Could you check a few things on this model? Use its own coordinates, in mm. A direction names the side the tool comes from. Round coordinates to 2 decimals unless told otherwise and drop trailing zeros. Write each loop counter-clockwise with the first axis right and the second up, starting at its lowest first coordinate (ties: lowest second). Pieces come first, ordered by that corner, then holes. Notation, with made-up numbers: (-8.5, -8.75) -> (-0.5, -8.75) arc R11 ccw to (-0.5, 2.25) -> close; hole circle Ø6 at (-37.75, 76.25). An arc over 180 degrees is marked (long way). Answer in a Markdown table with one row per item.
from build123d import *

# Parameters (mm, degrees)
SKETCH1_W           = 144
SKETCH1_H           = 51
BOSS_EXTRUDE1_DEPTH = 3
BOSS_EXTRUDE2_START = -3
SKETCH2_W           = 144
SKETCH2_H           = 51
SKETCH2_W_2         = 139
SKETCH2_H_2         = 46
BOSS_EXTRUDE2_DEPTH = 16
BOSS_EXTRUDE3_DEPTH = 16.5
SKETCH4_R           = 2
SKETCH4_R_2         = 1.5
CUT_EXTRUDE1_DEPTH  = 84.009035653


with BuildPart() as part:
    # Sketch1 → Boss-Extrude1 (new body)
    with BuildSketch(Plane(origin=(0, 0, 0), x_dir=(1, 0, 0), z_dir=(0, 1, 0))):
        Rectangle(SKETCH1_W, SKETCH1_H)
    extrude(amount=BOSS_EXTRUDE1_DEPTH)

    # Sketch2 → Boss-Extrude2 (add)
    with BuildSketch(Plane(origin=(0, 3, 0), x_dir=(1, 0, 0), z_dir=(0, 1, 0)).offset(BOSS_EXTRUDE2_START)):
        Rectangle(SKETCH2_W, SKETCH2_H)
        Rectangle(SKETCH2_W_2, SKETCH2_H_2, mode=Mode.SUBTRACT)
    extrude(amount=BOSS_EXTRUDE2_DEPTH)

    # Sketch3 → Boss-Extrude3 (add)
    with BuildSketch(Plane(origin=(0, 16, 0), x_dir=(1, 0, 0), z_dir=(0, 1, 0))):
        Polygon((-72, 25.5), (-72, 12.5), (-69.5, 12.5), (-69.5, 23), (-47, 23), (-47, 25.5), align=None)
        Polygon((47, 25.5), (72, 25.5), (72, 12.5), (69.5, 12.5), (69.5, 23), (47, 23), align=None)
        Polygon((72, -25.5), (72, -12.5), (69.5, -12.5), (69.5, -23), (47, -23), (47, -25.5), align=None)
        Polygon((-47, -25.5), (-72, -25.5), (-72, -12.5), (-69.5, -12.5), (-69.5, -23), (-47, -23), align=None)
    extrude(amount=BOSS_EXTRUDE3_DEPTH)

    # Sketch4 → Cut-Extrude1 (cut, through all)
    with BuildSketch(Plane.XZ):
        with Locations(Location((-45, -13, 0), (0, 0, 270))):
            Circle(SKETCH4_R)
        with Locations(Location((-45, 13, 0), (0, 0, 270))):
            Circle(SKETCH4_R)
        with Locations(Location((45, 13, 0), (0, 0, 270))):
            Circle(SKETCH4_R)
        with Locations(Location((45, -13, 0), (0, 0, 270))):
            Circle(SKETCH4_R)
        with Locations(Location((-50, -0.45, 0), (0, 0, 270))):
            Circle(SKETCH4_R_2)
        with Locations(Location((50, -0.45, 0), (0, 0, 270))):
            Circle(SKETCH4_R_2)
    extrude(amount=-CUT_EXTRUDE1_DEPTH, mode=Mode.SUBTRACT)


solid = part.part
1) Imagine slicing it at A-A, the plane x = -45. Please give me the cut outline in (y, z).
Findings:
| item | result |
|---|---|
| outline | (0, -25.5) -> (16, -25.5) -> (16, -23) -> (3, -23) -> (3, -15) -> (0, -15) -> close; (0, -11) -> (3, -11) -> (3, 11) -> (0, 11) -> close; (0, 15) -> (3, 15) -> (3, 23) -> (16, 23) -> (16, 25.5) -> (0, 25.5) -> close |
2) Imagine slicing it at D-D, the plane x = 50. Please give me the cut outline in (y, z).
Findings:
| item | result |
|---|---|
| outline | (0, -25.5) -> (32.5, -25.5) -> (32.5, -23) -> (3, -23) -> (3, -1.95) -> (0, -1.95) -> close; (0, 1.05) -> (3, 1.05) -> (3, 23) -> (32.5, 23) -> (32.5, 25.5) -> (0, 25.5) -> close |
3) Please list where these lines run through material, in increasing order: line 1 (X direction, y = 1.2, z = -13); line 2 (X direction, y = 1.8, z = -0.45); line 3 (X direction, y = 7.5, z = -9).
Findings:
| item | result |
|---|---|
| line 1 | x = -72 to -47, -43 to 43, 47 to 72 |
| line 2 | x = -72 to -51.5, -48.5 to 48.5, 51.5 to 72 |
| line 3 | x = -72 to -69.5, 69.5 to 72 |
4) For pin 1 (23 mm diameter, centred on x = -28, z = -9.5, fed in from +Y); pin 2 (0.8 mm diameter, centred on x = 17, z = 24.5, fed in from +Y), each with a flat end and sliding along its axis, tell me the tip position at first contact or that it passes through.
Findings:
| item | result |
|---|---|
| pin 1 | stops at y = 3 |
| pin 2 | stops at y = 16 |
5) For faces 5 (the face through (-51.464, 1.479, -0.125)), 6 (the face through (-1, 14, 23)), 7 (the face through (-71, 24, -12.5)), 8 (the face through (-47, 24, 24)), which set-ups out of +Z, -Z, +X, -X, +Y, -Y let a thin tool reach every point of the face, with its end or its side?
Findings:
| item | result |
|---|---|
| face 5 | +Y, -Y |
| face 6 | +Y |
| face 7 | +X, -X, +Y |
| face 8 | +Z, -Z, +Y |
6) Thinking about a two-plate mould opening in X: for faces 1 (the face through (-47, 24, -24)), 2 (the face through (-1, 16, -24)), 3 (the face through (-63.1, 32.5, 23.3)), 4 (the face through (72, 12, 0)), which applies, +X half, -X half, draft (parallel to the pull), parting line (faces both ways), or undercut?
Findings:
| item | result |
|---|---|
| face 1 | undercut |
| face 2 | undercut |
| face 3 | draft |
| face 4 | +X half |
7) Imagine slicing it at B-B, the plane z = -0.45. Please give me the cut outline in (x, y).
Findings:
| item | result |
|---|---|
| outline | (-72, 0) -> (-51.5, 0) -> (-51.5, 3) -> (-69.5, 3) -> (-69.5, 16) -> (-72, 16) -> close; (-48.5, 0) -> (48.5, 0) -> (48.5, 3) -> (-48.5, 3) -> close; (51.5, 0) -> (72, 0) -> (72, 16) -> (69.5, 16) -> (69.5, 3) -> (51.5, 3) -> close |
8) Imagine slicing it at C-C, the plane y = 27. Please give me the cut outline in (x, z).
Findings:
| item | result |
|---|---|
| outline | (-72, -25.5) -> (-47, -25.5) -> (-47, -23) -> (-69.5, -23) -> (-69.5, -12.5) -> (-72, -12.5) -> close; (-72, 12.5) -> (-69.5, 12.5) -> (-69.5, 23) -> (-47, 23) -> (-47, 25.5) -> (-72, 25.5) -> close; (47, -25.5) -> (72, -25.5) -> (72, -12.5) -> (69.5, -12.5) -> (69.5, -23) -> (47, -23) -> close; (47, 23) -> (69.5, 23) -> (69.5, 12.5) -> (72, 12.5) -> (72, 25.5) -> (47, 25.5) -> close |
